Can you work these out from the drawing? Everything is in mm from the part's minimum corner. Coordinates: 2 decimals unless noted, no trailing zeros. Write each loop counter-clockwise with the first axis right and the second up, starting at its lowest first coordinate (ties: lowest second). Pieces come first, ordered by that corner, then holes.
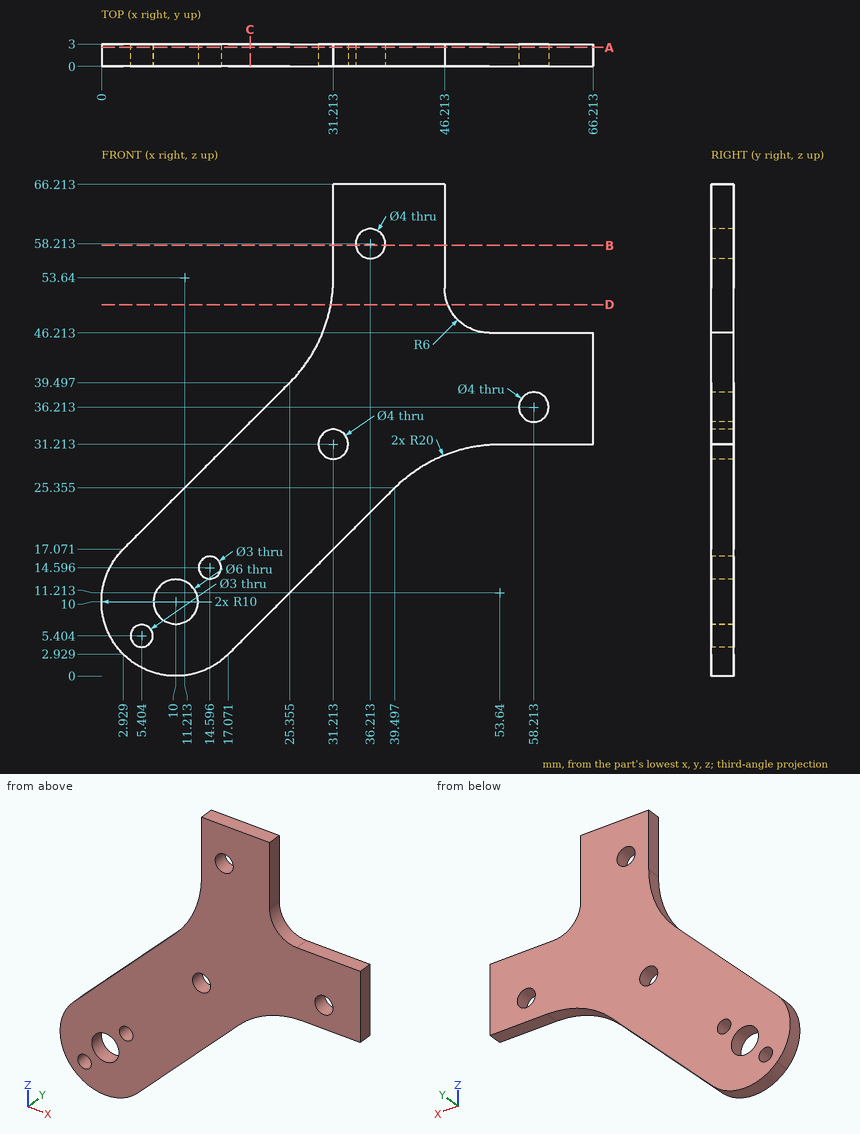
1. If I drill on line 1 (Z direction, x = 58, y = 0.2) (1 decimal); line 2 (Z direction, x = 33, y = 2.1) (1 decimal); line 3 (Z direction, x = 55, y = 2.7), over which ranges is the centre line in solid material (lowest first)?
2. For pin 1 Ø1.5 at (y, z) = (1, 60.5) entering from +X; pin 2 Ø2.5 at (x, z) = (5.4, 5.4) entering from +Y; pin 3 Ø1.5 at (x, y) = (57, 2) entering from +Z, each with a flat end and sliding along its axis, tell me the tip position at first contact or that it passes through.
3. I want a section at C-C (x = 20). List the corners of the cut face in (y, z) for me.
4. I want a section at D-D (z = 50). List the corners of the cut face in (x, y) for me.
5. I want a section at B-B (z = 58). List the corners of the cut face in (x, y) for me (1 decimal).
6. I want a section at A-A (y = 2.55). State how many separate pieces and enclosed holes the cut face has, then the cut area to 3 significant figures.
Response values:
1. line 1: z = 31.2 to 34.2, 38.2 to 46.2
1. line 2: z = 18.9 to 30.3, 32.1 to 66.2
1. line 3: z = 31.21 to 46.21
2. pin 1: stops at x = 46.21
2. pin 2: passes through
2. pin 3: stops at z = 46.21
3. outline: (0, 5.86) - (3, 5.86) - (3, 34.14) - (0, 34.14) - close
4. outline: (30.88, 0) - (46.64, 0) - (46.64, 3) - (30.88, 3) - close
5. outline: (31.2, 0) - (34.2, 0) - (34.2, 3) - (31.2, 3) - close; (38.2, 0) - (46.2, 0) - (46.2, 3) - (38.2, 3) - close
6. separate pieces: 1
6. enclosed holes: 6
6. area: 1,630 mm2
